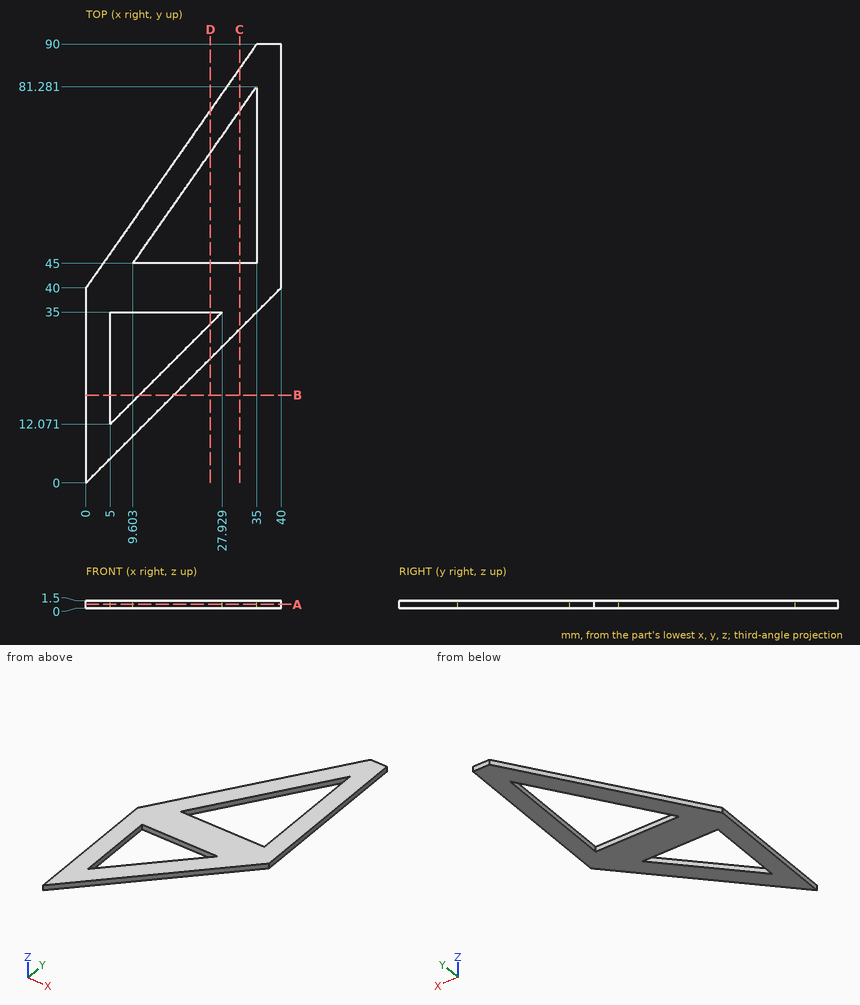
The drawing under review shows one solid part. Ordinate dimensions are in mm from its lowest x, y, z. Coordinates: 2 decimals unless noted, no trailing zeros. Write each loop counter-clockwise with the first axis right and the second up, starting at its lowest first coordinate (ties: lowest second). Pieces come first, ordered by that corner, then holes. Notation, with made-up numbers: M 56.25,70.25 L 92.25,70.25 A13 cw 92.25,83.25 Z; hole C 37.25,68 d11. An arc over 180 degrees is marked long. Answer as a JSON object with one key per item and string values.
Item 1: Add section C-C, the plane x = 31.5. Give the boundary of the cut face in (y, z).
Outcome:
{"outline": "M 31.5,0 L 45,0 L 45,1.5 L 31.5,1.5 Z; M 76.28,0 L 85,0 L 85,1.5 L 76.28,1.5 Z"}
Item 2: Add section B-B, the plane y = 18. Give the boundary of the cut face in (x, z).
Outcome:
{"outline": "M 0,0 L 5,0 L 5,1.5 L 0,1.5 Z; M 10.93,0 L 18,0 L 18,1.5 L 10.93,1.5 Z"}
Item 3: Add section A-A, the plane z = 0.8. Give the boundary of the cut face in (x, y).
Outcome:
{"outline": "M 0,0 L 40,40 L 40,90 L 35,90 L 0,40 Z; hole M 5,12.07 L 27.93,35 L 5,35 Z; hole M 9.6,45 L 35,45 L 35,81.28 Z"}
Item 4: Wall thickness on probe 1 along Y at (x, z) = (18, 1.4) (1 decimal); probe 2 along Y at (x, z) = (17, 1) (1 decimal); probe 3 along X at (y, z) = (69.5, 0.3): over which ranges is each line inside the solid? List them lowest first.
Outcome:
{"probe 1": "18 to 25.1, 35 to 45, 57 to 65.7", "probe 2": "17 to 24.1, 35 to 45, 55.6 to 64.3", "probe 3": "20.65 to 26.75, 35 to 40"}
Item 5: Insertion check: pin 1 Ø0.8 at (y, z) = (58.5, 0.5) entering from -X; pin 2 Ø0.8 at (y, z) = (26.5, 0.5) entering from +X. Each pin has a flat end and moves straight along its axis. Give the tip position at first contact, or say it passes through.
Outcome:
{"pin 1": "x = 12.67", "pin 2": "x = 26.9"}
Item 6: Add section D-D, the plane x = 25.5. Give the boundary of the cut face in (y, z).
Outcome:
{"outline": "M 25.5,0 L 32.57,0 L 32.57,1.5 L 25.5,1.5 Z; M 35,0 L 45,0 L 45,1.5 L 35,1.5 Z; M 67.71,0 L 76.43,0 L 76.43,1.5 L 67.71,1.5 Z"}
